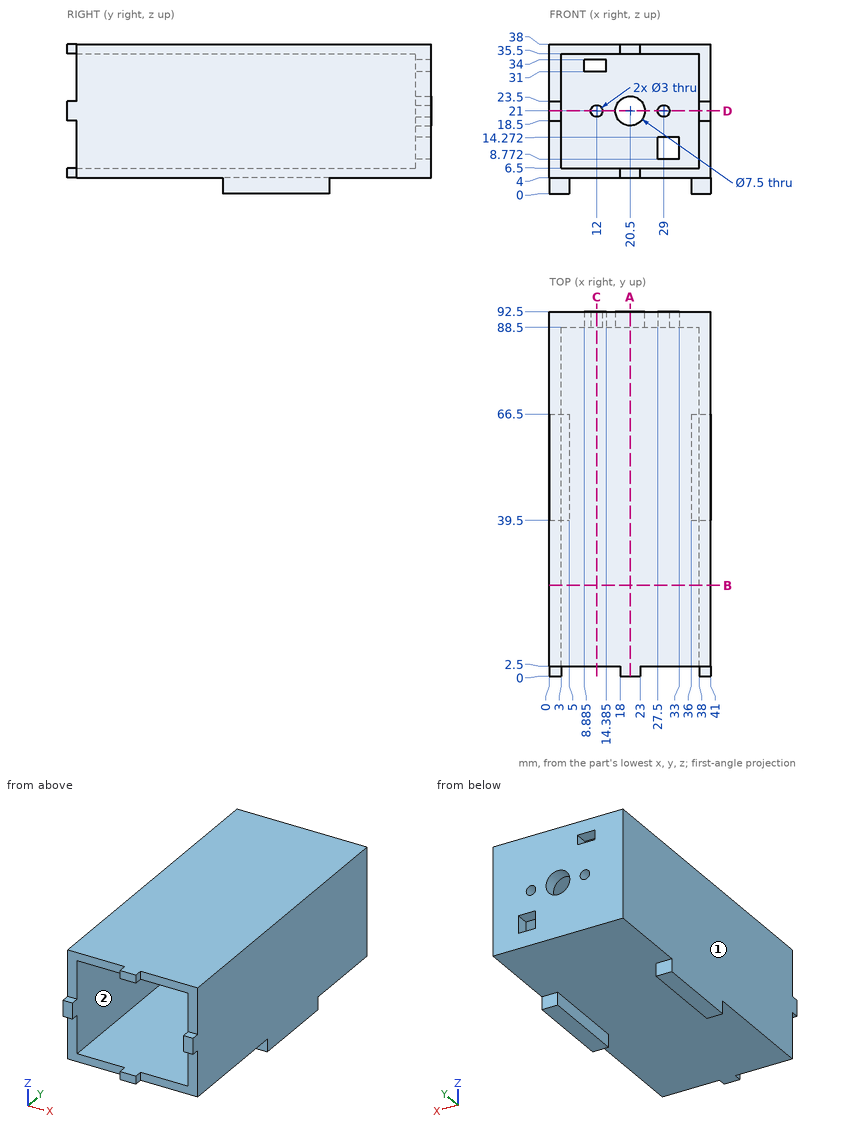
Design review of the part shown in the three views and the two pictorial views. Dimensions are in mm from the part's minimum x, y and z. A direction names the side the tool comes from. Give positions to 0.01 mm unless a question says otherwise; leave off trailing zeros. Write each loop counter-clockwise with the first axis right and the second up, starting at its lowest first coordinate (ties: lowest second). Pieces come first, ordered by that corner, then holes. Notation, with made-up numbers: M 76.5,67 L 115.5,67 A12 cw 115.5,72 Z; hole C -8,53 d9. An arc over 180 degrees is marked long. One line per item, written item: value.
1) Take a section at B-B, the plane y = 23. Write out the cut boundary in (x, z), then the cut area to 3 significant figures.
Results are:
outline: M 0,4 L 41,4 L 41,38 L 0,38 Z; hole M 3,6.5 L 38,6.5 L 38,35.5 L 3,35.5 Z
area: 379 mm²
2) Take a section at A-A, the plane x = 20.5. Write out the cut boundary in (y, z).
Results are:
outline: M 0,4 L 92.5,4 L 92.5,17.25 L 88.5,17.25 L 88.5,6.5 L 0,6.5 Z; M 0,35.5 L 88.5,35.5 L 88.5,24.75 L 92.5,24.75 L 92.5,38 L 0,38 Z
3) For the marked faces 1 and 2, list the 3-axis set-ups (+Z, -Z, +X, -X, +Y, -Y) from which the entire face can be reached by the end or side of a thin tool; tool diameter is ignored.
Results are:
face 1: +Z, -Z, -X, +Y, -Y
face 2: -Y
4) For line 1 (Z direction, x = 29, y = 89.35); line 2 (Z direction, x = 30, y = 67); line 3 (X direction, y = 45, z = 10.5), list the stretches that pass through material, from the lowest coordinate up. Write a range as from..to.
Results are:
line 1: z = 4..8.77, 14.27..19.5, 22.5..38
line 2: z = 4..6.5, 35.5..38
line 3: x = 0..3, 38..41
5) Take a section at C-C, the plane x = 12. Write out the cut boundary in (y, z), then the cut area to 3 significant figures.
Results are:
outline: M 2.5,4 L 92.5,4 L 92.5,19.5 L 88.5,19.5 L 88.5,6.5 L 2.5,6.5 Z; M 2.5,35.5 L 88.5,35.5 L 88.5,34 L 92.5,34 L 92.5,38 L 2.5,38 Z; M 88.5,22.5 L 92.5,22.5 L 92.5,31 L 88.5,31 Z
area: 542 mm²
6) For P1, Ø12.5, axis at x = 22, y = 61.5, coming from the -Z side; P2, Ø14.5, axis at x = 24.5, z = 16.5, coming from the -Y side; P3, Ø2, axis at x = 2.5, z = 1.5, coming from the +Y side, all flat-tipped, find the tip position at first contact; note any pin that passes through.
Results are:
P1: stops at z = 4
P2: stops at y = 88.5
P3: stops at y = 66.5
7) Take a section at D-D, the plane z = 21. Write out the cut boundary in (x, y), then the cut area to 3 significant figures.
Results are:
outline: M 0,0 L 3,0 L 3,88.5 L 10.5,88.5 L 10.5,92.5 L 0,92.5 Z; M 13.5,88.5 L 16.75,88.5 L 16.75,92.5 L 13.5,92.5 Z; M 24.25,88.5 L 27.5,88.5 L 27.5,92.5 L 24.25,92.5 Z; M 30.5,88.5 L 38,88.5 L 38,0 L 41,0 L 41,92.5 L 30.5,92.5 Z
area: 641 mm²
